Geometry: see drawing. Coordinates: mm, zero at the bounding-box minimum. Give positions to 0.01 mm unless a question says otherwise; leave off trailing zeros. Loops run counter-clockwise (first coordinate to the right, second up) from the corner with the lowest first, then second, coordinate; pieces in that order, holes last. Notation, with made-up numbers: (70, 17.5) - (127, 17.5) arc R32 cw to (127, 49.5) - close; hole circle Ø3 at (6.25, 69). An arc over 180 degrees is marked (long way). Use CSV: the item, a comma, the result in double quotes. Start each with the question number.
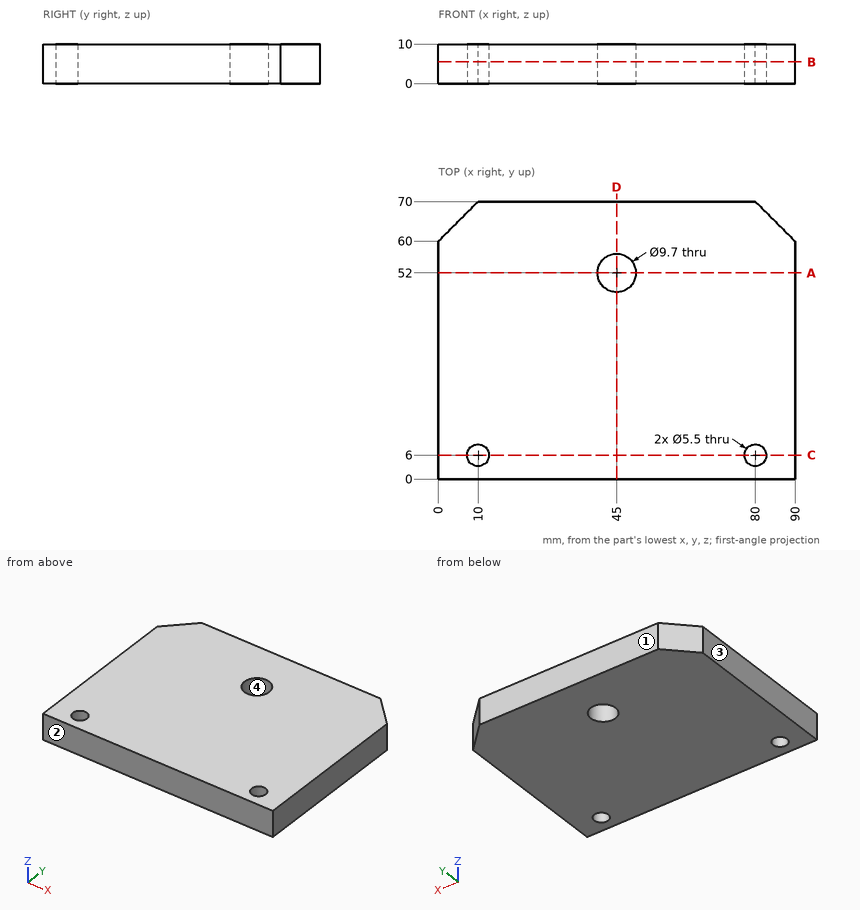
Item 1: Ray query, probe 1 along X at (y, z) = (6, 5.5); probe 2 along Y at (x, z) = (45, 5.5); probe 3 along Y at (x, z) = (10, 2.75). Return the intervals inside material, ascending.
Item 2: Section D-D (x = 45). Output: boundary loops of the cut face in (y, z).
Item 3: Section C-C (y = 6). Output: boundary loops of the cut face in (x, z).
Item 4: Pin query (flat end, axial travel): pin 1 Ø9 at (x, y) = (80, 6) entering from +Z; pin 2 Ø3 at (y, z) = (62, 1.5) entering from +X. Return the tip coordinate at first contact, or that it passes through.
Item 5: Section B-B (z = 5.5). Output: boundary loops of the cut face in (x, y), plus the area to 3 significant figures.
Item 6: Section A-A (y = 52). Output: boundary loops of the cut face in (x, z).
Item 7: Mould query, pull axis Y, two halves, no side actions, for the marked faces 1, 2, 3 and 4. Classes: pulls with the +Y half, pulls with the -Y half, needs draft (parallel to the pull), parting line crosses it, or undercut.
Outcome:
1,probe 1,"x = 0 to 7.25, 12.75 to 77.25, 82.75 to 90"
1,probe 2,"y = 0 to 47.15, 56.85 to 70"
1,probe 3,"y = 0 to 3.25, 8.75 to 70"
2,outline,"(0, 0) - (47.15, 0) - (47.15, 10) - (0, 10) - close; (56.85, 0) - (70, 0) - (70, 10) - (56.85, 10) - close"
3,outline,"(0, 0) - (7.25, 0) - (7.25, 10) - (0, 10) - close; (12.75, 0) - (77.25, 0) - (77.25, 10) - (12.75, 10) - close; (82.75, 0) - (90, 0) - (90, 10) - (82.75, 10) - close"
4,pin 1,"stops at z = 10"
4,pin 2,"stops at x = 89.5"
5,outline,"(0, 0) - (90, 0) - (90, 60) - (80, 70) - (10, 70) - (0, 60) - close; hole circle Ø5.5 at (10, 6); hole circle Ø9.7 at (45, 52); hole circle Ø5.5 at (80, 6)"
5,area,"6,080 mm2"
6,outline,"(0, 0) - (40.15, 0) - (40.15, 10) - (0, 10) - close; (49.85, 0) - (90, 0) - (90, 10) - (49.85, 10) - close"
7,face 1,"pulls with the +Y half"
7,face 2,"pulls with the -Y half"
7,face 3,"needs draft"
7,face 4,"undercut"
